```python
from build123d import *

# Parameters (mm, degrees)
F1_W      = 75
F1_H      = 65
F2_DEPTH  = 10
F3_R      = 5.5
F4_DEPTH  = 7
F5_R      = 4.75
F6_DEPTH  = 5.5
F7_R      = 3.5
F8_DEPTH  = 25
F9_R      = 2.75
F10_DEPTH = 25
F11_R     = 2
F11_R_2   = 2.5
F12_DEPTH = 25
F13_SIZE  = 1


with BuildPart() as f2:
    # F1 (on face) → F2 (new body)
    with BuildSketch(Plane.XY):
        Rectangle(F1_W, F1_H)
    extrude(amount=F2_DEPTH)

    # F3 (on face) → F4 (cut)
    with BuildSketch(Plane.XY):
        with Locations((-8, 22)):
            Circle(F3_R)
        with Locations((-8, -22)):
            Circle(F3_R)
    extrude(amount=F4_DEPTH, mode=Mode.SUBTRACT)

    # F5 (on face) → F6 (cut)
    with BuildSketch(Plane.XY):
        with Locations((-29.5, 22)):
            Circle(F5_R)
        with Locations((-29.5, -17)):
            Circle(F5_R)
    extrude(amount=F6_DEPTH, mode=Mode.SUBTRACT)

    # F7 (on face) → F8 (cut)
    with BuildSketch(Plane.XY):
        with Locations((-8, -22)):
            Circle(F7_R)
        with Locations((-8, 22)):
            Circle(F7_R)
    extrude(amount=F8_DEPTH, mode=Mode.SUBTRACT)

    # F9 (on face) → F10 (cut)
    with BuildSketch(Plane.XY):
        with Locations((-29.5, -17)):
            Circle(F9_R)
        with Locations((-29.5, 22)):
            Circle(F9_R)
    extrude(amount=F10_DEPTH, mode=Mode.SUBTRACT)

    # F11 (on face) → F12 (cut)
    with BuildSketch(Plane.XY):
        with Locations((-19.5, -27.5)):
            Circle(F11_R)
        with Locations((-19.5, 12.5)):
            Circle(F11_R_2)
        with Locations((25.5, -27.5)):
            Circle(F11_R)
        with Locations((25.5, 12.5)):
            Circle(F11_R_2)
    extrude(amount=F12_DEPTH, mode=Mode.SUBTRACT)

    # F13
    f13_edges = [f2.edges().sort_by_distance(p)[0] for p in [
        (-37.5, 32.5, 5),
        (-37.5, -32.5, 5),
        (37.5, -32.5, 5),
        (37.5, 32.5, 5),
    ]]
    chamfer(f13_edges, length=F13_SIZE)


solid = f2.part
```
Here's how the part is built. I have some questions about the finished solid (model axes, mm). A direction names the side the tool comes from. Round coordinates to 2 decimals unless told otherwise and drop trailing zeros. Write each loop counter-clockwise with the first axis right and the second up, starting at its lowest first coordinate (ties: lowest second). Pieces come first, ordered by that corner, then holes.
Q1. Please list where these lines run through material, in increasing order: probe 1 along Y at (x, z) = (-29.5, 6.5); probe 2 along X at (y, z) = (22, 8.25); probe 3 along Y at (x, z) = (-19.5, 7).
Q2. If we section it at C-C on z = 8.75: Give the number of separate pieces and of enclosed holes in the cut face, plus the area to 3 significant figures.
Q3. If we mould it in two halves opening along X, with no side actions, what happens to faces 1 (the flat face through (-37.5, 0, 5)), 2 (the flat face through (-4, -22, 7)), 3 (the flat face through (-1, 0, 0))? For each: +X half, -X half, draft (parallel to the pull), parting line (faces both ways), or undercut.
Q4. If we section it at D-D on y = -23: Write out the boundary of the cut face in (x, z), plus the area to 3 significant figures.
Q5. If we section it at A-A on y = 12.5: Write out the boundary of the cut face in (x, z).
Q6. Will these pins go through, and if not, where does the flat tip stop? P1, Ø6.5, axis at x = -29.5, y = 22, coming from the +Z side; P2, Ø2.5, axis at x = -19.5, y = -27.5, coming from the -Z side; P3, Ø5.5, axis at x = -6.5, y = 21.5, coming from the -Z side.
Q7. If we section it at B-B on x = -8: Write out the boundary of the cut face in (y, z).
Q8. Which directions (+Z, -Z, +X, -X, +Y, -Y) give clear straight access to the entire face, cutting with the end or side of a thin tool? Please do faces 4 (the flat face through (37.5, 0, 5)), 5 (the flat face through (-4, 22, 7)).
Answer below:
1. probe 1: y = -32.5 to -19.75, -14.25 to 19.25, 24.75 to 32.5
1. probe 2: x = -37.5 to -32.25, -26.75 to -11.5, -4.5 to 37.5
1. probe 3: y = -32.5 to -29.5, -25.5 to 10, 15 to 32.5
2. separate pieces: 1
2. enclosed holes: 8
2. area: 4,680 mm2
3. face 1: -X half
3. face 2: undercut
3. face 3: draft
4. outline: (-37.5, 0) - (-13.41, 0) - (-13.41, 7) - (-11.35, 7) - (-11.35, 10) - (-37.5, 10) - close; (-4.65, 7) - (-2.59, 7) - (-2.59, 0) - (37.5, 0) - (37.5, 10) - (-4.65, 10) - close
4. area: 654 mm2
5. outline: (-37.5, 0) - (-22, 0) - (-22, 10) - (-37.5, 10) - close; (-17, 0) - (23, 0) - (23, 10) - (-17, 10) - close; (28, 0) - (37.5, 0) - (37.5, 10) - (28, 10) - close
6. P1: stops at z = 10
6. P2: passes through
6. P3: stops at z = 7
7. outline: (-32.5, 0) - (-27.5, 0) - (-27.5, 7) - (-25.5, 7) - (-25.5, 10) - (-32.5, 10) - close; (-18.5, 7) - (-16.5, 7) - (-16.5, 0) - (16.5, 0) - (16.5, 7) - (18.5, 7) - (18.5, 10) - (-18.5, 10) - close; (25.5, 7) - (27.5, 7) - (27.5, 0) - (32.5, 0) - (32.5, 10) - (25.5, 10) - close
8. face 4: +Z, -Z, +X, +Y, -Y
8. face 5: -Z
